Could you check a few things on this model? Use its own coordinates, in mm. Face numbers are marked on the shaded views. A direction names the side the tool comes from. Give positions to 0.01 mm unless a question says otherwise; leave off trailing zeros. Order: outer loops, then holes, each group sorted by start corner. A loop starts at its lowest first (then second) coordinate and runs counter-clockwise, first axis right, second up. Notation, with made-up numbers: (28, 36.25) - (85, 36.25) arc R20 ccw to (85, 52.25) - close; hole circle Ø10 at (-32, 52.25). An arc over 180 degrees is marked (long way). One line per question, with ' | ' between items. Start each with the question number.
1. Imagine slicing it at B-B (x = 32). Please give me the cut outline in (y, z), and give its area (3 significant figures).
2. I need wall thicknesses on probe 1 along Y at (x, z) = (-2, 3.75); probe 2 along X at (y, z) = (18, 1.2); probe 3 along X at (y, z) = (-19, 0.7). Which ranges of each line are inside material? Lowest first, please. Write a range as from..to.
3. Imagine slicing it at A-A (y = 17.5). Please give me the cut outline in (x, z), and give its area (3 significant figures).
4. Which directions (+Z, -Z, +X, -X, +Y, -Y) give clear straight access to the entire face, cutting with the end or side of a thin tool? Please do the marked faces 1 and 2.
5. Imagine slicing it at D-D (y = -32.5). Please give me the cut outline in (x, z), and give its area (4 significant figures).
6. For P1, Ø1.3, axis at y = -30, z = 1.5, coming from the -X side; P2, Ø0.9, axis at y = 17, z = 2, coming from the -X side; P3, Ø1, axis at y = -26, z = 1.5, coming from the -X side, each with a flat end and sliding along its axis, tell me the tip position at first contact or that it passes through.
7. Imagine slicing it at C-C (z = 1.35). Give the number of separate pieces and of enclosed holes in the cut face, and give its area (3 significant figures).
8. If we mould it in two halves opening along Y, with no side actions, what happens to the marked faces 3, 4 and 5? For each: released by +Y, released by -Y, zero draft, split by the parting line, or undercut.
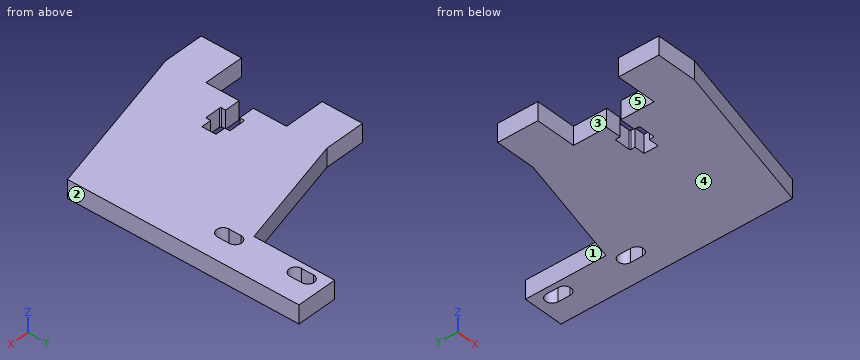
```python
from build123d import *

# Parameters (mm, degrees)
BOSS_EXTRUDE1_DEPTH = 4.5
SCREW_CUTOUT_DEPTH  = 60.718087712
CUT_EXTRUDE2_DEPTH  = 60.718087712


with BuildPart() as part:
    # Sketch1 → Boss-Extrude1 (new body)
    with BuildSketch(Plane.XY):
        Polygon((29, 2.5), (0, -5), (-10, -5), (-10, -15), (0, -15), (0, -35), (-10, -35), (-10, -45), (0, -45), (39, -34.913793103), (39, 22.5), (29, 22.5), align=None)
    extrude(amount=BOSS_EXTRUDE1_DEPTH)

    # Sketch2 → screw-cutout (cut, through all)
    with BuildSketch(Plane.XY.offset(4.5)):
        with BuildLine():
            Line((0, -26.75), (0, -23.25))
            Line((0, -23.25), (3.8, -23.25))
            Line((3.8, -23.25), (3.8, -22.25))
            ThreePointArc((3.8, -22.25), (3.873223305, -22.073223305), (4.05, -22))
            Line((4.05, -22), (7.75, -22))
            ThreePointArc((7.75, -22), (7.926776695, -22.073223305), (8, -22.25))
            Line((8, -22.25), (8, -23.25))
            Line((8, -23.25), (10.5, -23.25))
            Line((10.5, -23.25), (10.5, -26.75))
            Line((10.5, -26.75), (8, -26.75))
            Line((8, -26.75), (8, -27.75))
            ThreePointArc((8, -27.75), (7.926776695, -27.926776695), (7.75, -28))
            Line((7.75, -28), (4.05, -28))
            ThreePointArc((4.05, -28), (3.873223305, -27.926776695), (3.8, -27.75))
            Line((3.8, -27.75), (3.8, -26.75))
            Line((3.8, -26.75), (0, -26.75))
        make_face()
    extrude(amount=-SCREW_CUTOUT_DEPTH, mode=Mode.SUBTRACT)

    # Sketch3 → Cut-Extrude2 (cut, through all)
    with BuildSketch(Plane.XY.offset(4.5)):
        with BuildLine():
            Line((33.6, 18.5), (33.6, 15.5))
            ThreePointArc((33.6, 15.5), (32, 13.9), (30.4, 15.5))
            Line((30.4, 15.5), (30.4, 18.5))
            ThreePointArc((30.4, 18.5), (32, 20.1), (33.6, 18.5))
        make_face()
        with BuildLine():
            Line((33.6, 0.5), (33.6, -2.5))
            ThreePointArc((33.6, -2.5), (32, -4.1), (30.4, -2.5))
            Line((30.4, -2.5), (30.4, 0.5))
            ThreePointArc((30.4, 0.5), (32, 2.1), (33.6, 0.5))
        make_face()
    extrude(amount=-CUT_EXTRUDE2_DEPTH, mode=Mode.SUBTRACT)


solid = part.part
```
Results found:
1) outline: (-36.72, 0) - (-4.1, 0) - (-4.1, 4.5) - (-36.72, 4.5) - close; (2.1, 0) - (13.9, 0) - (13.9, 4.5) - (2.1, 4.5) - close; (20.1, 0) - (22.5, 0) - (22.5, 4.5) - (20.1, 4.5) - close | area: 211 mm2
2) probe 1: y = -45..-35, -15..-5 | probe 2: x = 29..30.4, 33.6..39 | probe 3: x = 0..39
3) outline: (29, 0) - (30.4, 0) - (30.4, 4.5) - (29, 4.5) - close; (33.6, 0) - (39, 0) - (39, 4.5) - (33.6, 4.5) - close | area: 30.6 mm2
4) face 1: +Z, -Z, -X, +Y | face 2: +Z, -Z, +X, +Y, -Y
5) outline: (0, 0) - (39, 0) - (39, 4.5) - (0, 4.5) - close | area: 175.5 mm2
6) P1: stops at x = 0 | P2: stops at x = 29 | P3: stops at x = 10.5
7) separate pieces: 1 | enclosed holes: 2 | area: 1,860 mm2
8) face 3: undercut | face 4: zero draft | face 5: undercut
